```python
from build123d import *

# Parameters (mm, degrees)
SKICA1_W                      = 54.3
SKICA1_H                      = 104.3
P_IDAT_VYSUNUT_M1_DEPTH       = 0.9
ZAOBLIT1_R                    = 2
SKICA2_R                      = 1.1
ODEBRAT_VYSUNUT_M1_DEPTH      = 0.9
P_IDAT_VYSUNUT_M2_DEPTH       = 6
ODEBRAT_VYSUNUT_M2_DEPTH      = 118.332817234
ODEBRAT_VYSUNUT_M2_DEPTH_BACK = 118.332817234
SKICA4_R                      = 1.2
SKICA5_W                      = 6
SKICA5_H                      = 50.3
P_IDAT_VYSUNUT_M3_DEPTH       = 2


with BuildPart() as part:
    # Skica1 → Přidat vysunutím1 (new body)
    with BuildSketch(Plane.XY):
        with Locations((27.15, 52.15)):
            Rectangle(SKICA1_W, SKICA1_H)
    extrude(amount=P_IDAT_VYSUNUT_M1_DEPTH)

    # Zaoblit1
    zaoblit1_edges = [part.edges().sort_by_distance(p)[0] for p in [
        (0, 104.3, 0.45),
        (54.3, 104.3, 0.45),
        (54.3, 0, 0.45),
        (0, 0, 0.45),
    ]]
    fillet(zaoblit1_edges, radius=ZAOBLIT1_R)

    # Skica2 → Odebrat vysunutím1 (cut)
    with BuildSketch(Plane.XY.offset(0.9)):
        with Locations((5.15, 99)):
            Circle(SKICA2_R)
        with Locations((49.15, 99)):
            Circle(SKICA2_R)
        with Locations((5.15, 5.3)):
            Circle(SKICA2_R)
        with Locations((49.15, 5.3)):
            Circle(SKICA2_R)
    extrude(amount=-ODEBRAT_VYSUNUT_M1_DEPTH, mode=Mode.SUBTRACT)

    # Skica3 → Přidat vysunutím2 (add)
    with BuildSketch(Plane.XY.offset(0.9)):
        with BuildLine():
            Line((7, 92.3), (7, 77.3))
            ThreePointArc((7, 77.3), (4, 74.3), (1, 77.3))
            Line((1, 77.3), (1, 92.3))
            ThreePointArc((1, 92.3), (4, 95.3), (7, 92.3))
        make_face()
        with BuildLine():
            Line((53.3, 92.3), (53.3, 77.3))
            ThreePointArc((53.3, 77.3), (50.3, 74.3), (47.3, 77.3))
            Line((47.3, 77.3), (47.3, 92.3))
            ThreePointArc((47.3, 92.3), (50.3, 95.3), (53.3, 92.3))
        make_face()
        with BuildLine():
            Line((7, 27), (7, 12))
            ThreePointArc((7, 12), (4, 9), (1, 12))
            Line((1, 12), (1, 27))
            ThreePointArc((1, 27), (4, 30), (7, 27))
        make_face()
        with BuildLine():
            Line((53.3, 27), (53.3, 12))
            ThreePointArc((53.3, 12), (50.3, 9), (47.3, 12))
            Line((47.3, 12), (47.3, 27))
            ThreePointArc((47.3, 27), (50.3, 30), (53.3, 27))
        make_face()
    extrude(amount=P_IDAT_VYSUNUT_M2_DEPTH)

    # Skica4 → Odebrat vysunutím2 (cut, two sides: drawn at the far end of the back side and taken through both)
    with BuildSketch(Plane(origin=(53.3, 0, 0), x_dir=(0, 0, -1), z_dir=(1, 0, 0)).offset(-ODEBRAT_VYSUNUT_M2_DEPTH_BACK)):
        with Locations((-3.9, 84.8)):
            Circle(SKICA4_R)
    extrude(amount=ODEBRAT_VYSUNUT_M2_DEPTH + ODEBRAT_VYSUNUT_M2_DEPTH_BACK, mode=Mode.SUBTRACT)

    # Skica5 → Přidat vysunutím3 (add)
    with BuildSketch(Plane.XY.offset(0.9)):
        with Locations((4, 52.15)):
            Rectangle(SKICA5_W, SKICA5_H)
        with Locations((50.3, 52.15)):
            Rectangle(SKICA5_W, SKICA5_H)
    extrude(amount=P_IDAT_VYSUNUT_M3_DEPTH)


solid = part.part
```
Check sheet for the modelled part. Datum: model origin and axes. Units: mm. A direction names the side the tool comes from. Give positions to 0.01 mm unless a question says otherwise; leave off trailing zeros. Loops run counter-clockwise (first coordinate to the right, second up) from the corner with the lowest first, then second, coordinate; pieces in that order, holes last. Notation, with made-up numbers: (-17, 6.5) - (-8, 6.5) arc R35 ccw to (-8, 44.5) - close; hole circle Ø4 at (-24.5, 30). An arc over 180 degrees is marked (long way). One line per question, with ' | ' between items. Start each with the question number.
1. Material ranges on line 1 along Y through (x, z) = (49.15, 0.6); line 2 along X through (y, z) = (99, 0.35); line 3 along Y through (x, z) = (4.45, 3.9), recorded low to high. Write a range as [from, to].
2. Cross-section at B-B, the plane x = 49.15. Enter the section's corners in (y, z).
3. Gauge pin test, flat ends, axial feed: pin 1 Ø2 at (x, z) = (7, 4) entering from -Y; pin 2 Ø3 at (x, y) = (3, 41.5) entering from +Z; pin 3 Ø3 at (y, z) = (84.8, 3.9) entering from +X; pin 4 Ø2 at (y, z) = (84.8, 3.9) entering from -X. Record the tip position at first contact, or that the pin passes through.
4. Draft check along X on faces 4 (the cylindrical face through (3.9, 95.3, 3.9)), 5 (the flat face through (27, 53, 0)), 6 (the cylindrical face through (53.73, 103.7, 0.46)). Enter one of: released by +X, released by -X, zero draft, split by the parting line, or undercut.
5. Cross-section at D-D, the plane y = 48.5. Enter the section's corners in (x, z), plus the area to 3 significant figures.
6. Cross-section at C-C, the plane z = 3.9. Enter the section's corners in (x, y), plus the area to 3 significant figures.
7. Set-up check for faces 1 (the flat face through (1, 51.6, 2.5)), 2 (the cylindrical face through (50.2, 30, 4.9)), 3 (the flat face through (7, 52.7, 2.5)): record each of +Z, -Z, +X, -X, +Y, -Y from which the full face is reachable in a straight line by a thin tool's end or side.
8. Cross-section at A-A, the plane y = 5.3. Enter the section's corners in (x, z), plus the area to 3 significant figures.
Check result:
1) line 1: y = [0, 4.2], [6.4, 97.9], [100.1, 104.3] | line 2: x = [0, 4.05], [6.25, 48.05], [50.25, 54.3] | line 3: y = [9.03, 29.97], [74.33, 83.6], [86, 95.27]
2) outline: (0, 0) - (4.2, 0) - (4.2, 0.9) - (0, 0.9) - close; (6.4, 0) - (97.9, 0) - (97.9, 0.9) - (95.07, 0.9) - (95.07, 6.9) - (74.53, 6.9) - (74.53, 2.9) - (29.77, 2.9) - (29.77, 6.9) - (9.23, 6.9) - (9.23, 0.9) - (6.4, 0.9) - close; (100.1, 0) - (104.3, 0) - (104.3, 0.9) - (100.1, 0.9) - close; hole circle Ø2.4 at (84.8, 3.9)
3) pin 1: stops at y = 9.76 | pin 2: stops at z = 2.9 | pin 3: stops at x = 53.3 | pin 4: passes through
4) face 4: undercut | face 5: zero draft | face 6: released by +X
5) outline: (0, 0) - (54.3, 0) - (54.3, 0.9) - (53.3, 0.9) - (53.3, 2.9) - (47.3, 2.9) - (47.3, 0.9) - (7, 0.9) - (7, 2.9) - (1, 2.9) - (1, 0.9) - (0, 0.9) - close | area: 72.9 mm2
6) outline: (1, 12) arc R3 ccw to (7, 12) - (7, 27) arc R3 ccw to (1, 27) - close; (1, 77.3) arc R3 ccw to (7, 77.3) - (7, 83.6) - (1, 83.6) - close; (1, 86) - (7, 86) - (7, 92.3) arc R3 ccw to (1, 92.3) - close; (47.3, 12) arc R3 ccw to (53.3, 12) - (53.3, 27) arc R3 ccw to (47.3, 27) - close; (47.3, 77.3) arc R3 ccw to (53.3, 77.3) - (53.3, 83.6) - (47.3, 83.6) - close; (47.3, 86) - (53.3, 86) - (53.3, 92.3) arc R3 ccw to (47.3, 92.3) - close | area: 444 mm2
7) face 1: +Z, -X, +Y, -Y | face 2: +Z | face 3: +Z, +Y, -Y
8) outline: (0, 0) - (4.05, 0) - (4.05, 0.9) - (0, 0.9) - close; (6.25, 0) - (48.05, 0) - (48.05, 0.9) - (6.25, 0.9) - close; (50.25, 0) - (54.3, 0) - (54.3, 0.9) - (50.25, 0.9) - close | area: 44.9 mm2
